Check sheet for the modelled part. Datum: model origin and axes. Units: mm. Face numbers are marked on the shaded views. A direction names the side the tool comes from. Round coordinates to 2 decimals unless told otherwise and drop trailing zeros. Order: outer loops, then holes, each group sorted by start corner. A loop starts at its lowest first (then second) coordinate and runs counter-clockwise, first axis right, second up. Notation, with made-up numbers: (-14, -26) -> (1, -26) arc R27 ccw to (1, 7) -> close; hole circle Ø10 at (29.5, -27). An arc over 180 degrees is marked (long way). Use CSV: the item, a comma, the result in double quotes.
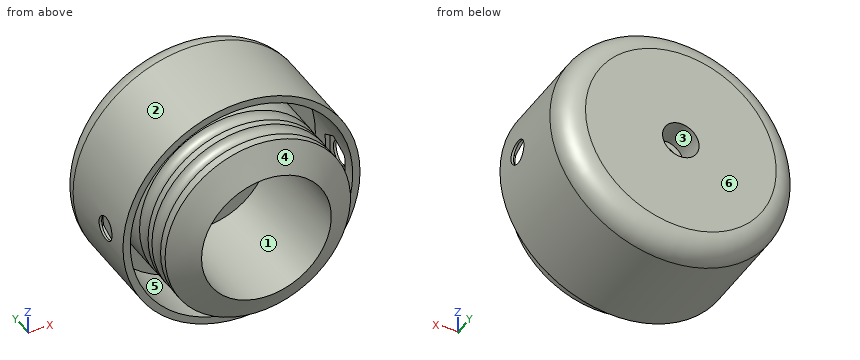
Autodesk Inventor part; units mm, degrees
ref_plane "Work Plane4" through (-32.48, 0, 0) normal (1, 0, 0) x (0, 1, 0)
ref_plane "Work Plane5" through (30.48, 0, 0) normal (1, 0, 0) x (0, 1, 0)
ref_plane "XZ Plane" through (0, 0, 0) normal (0, 1, 0) x (-1, 0, 0)
sketch "Sketch1" plane through (0, 0, 0) normal (0, 1, 0) x (-1, 0, 0)
  circle A0 centre (0, 0) radius 30.48
  circle A1 centre (0, 0) radius 32.48
  dimension "d0" = 60.96
  dimension "d2" = 2
extrude "Extrusion1" add sketch "Sketch1" along normal blind 19.05
sketch "Sketch2" plane through (0, 19.05, 0) normal (0, 1, 0) x (1, 0, 0)
  circle A0 centre (0, 0) radius 32.48
  circle A1 centre (0, 0) radius 32.48
extrude "Extrusion2" add sketch "Sketch2" along normal blind 12.7
fillet "Fillet1" radius 6.35 1 edges at (-32.48, 31.75, 0)
sketch "Sketch6" plane through (0, 31.75, 0) normal (0, 1, 0) x (1, 0, 0)
  circle A0 centre (0, 0) radius 3.302
  dimension "d15" = 6.604
extrude "Extrusion5" cut sketch "Sketch6" against normal up to surface (12.7 mm away)
sketch "Sketch10" plane through (0, 0, 0) normal (0, 0, 1) x (1, 0, 0)
  line L0 (-17.78, 19.05) -> (-17.78, -12.7)
  line L1 (-17.78, -12.7) -> (-25.4, -12.7)
  line L2 (-25.4, -12.7) -> (-25.4, 19.05)
  line L3 (-17.78, 19.05) -> (-25.4, 19.05)
  line L4 (-26.13, 31.75) -> (26.13, 31.75)
  line L5 (0, 31.75) -> (0, 0)
  line L6 (32.48, 0) -> (-32.48, 0)
  line L7 (-30.48, 0) -> (-30.48, 19.05)
  line L8 (-17.78, -12.7) -> (-25.4, -8.3006)
  line L9 (-30.48, 19.05) -> (30.48, 19.05)
  point P0 (-30.48, 0)
  point P1 (-25.4, 19.05)
  dimension "d29" = 7.62
  dimension "d33" = 30
  dimension "d42" = 25.4
  dimension "d89" = 31.75
revolve "Revolution2" add sketch "Sketch10" angle 360 about axis through (0, 31.75, 0) along (0, -1, 0) contours L0 L6 L2 L3 | L0 L8 L2 L6
sketch "Sketch11" plane through (0, 0, 0) normal (0, 0, 1) x (1, 0, 0)
  line L0 (25.4, -7.0306) -> (25.4, 25.4)
  circle A0 centre (26.3462, -3.81) radius 2.3813
  circle A1 centre (26.3462, 2.54) radius 2.3813
  line L1 (0, -11.43) -> (0, 31.75)
  line L2 (-26.13, 31.75) -> (26.13, 31.75)
  line L3 (26.3462, 2.54) -> (26.3462, -3.81)
  line L4 (30.48, 19.05) -> (30.48, 0)
  line L5 (30.48, 0) -> (29.972, 19.05)
  line L6 (29.972, 19.05) -> (29.972, 0)
  line L7 (-25.4, -5.08) -> (25.4, -5.08)
  line L8 (-17.78, -12.7) -> (17.78, -12.7)
  point P0 (0, 0)
  point P1 (25.4, -8.3006)
  point P2 (27.772, -0.6806)
  point P3 (17.78, -12.7)
  dimension "d36" = 6.35
  dimension "d37" = 4.7625
  dimension "d38" = 4.7625
  dimension "d43" = 26.3462
  dimension "d91" = 8.89
revolve "Revolution3" cut sketch "Sketch11" angle 360 about axis through (0, -11.43, 0) along (0, 1, 0) contours A0 L7 L0 | L0 A0 | L7 A0 L0 | A1 L0 | L0 A1
sketch "Sketch23" plane through (0, 31.75, 0) normal (0, 1, 0) x (1, 0, 0)
  circle A0 centre (0, 0) radius 5
  dimension "d103" = 10
extrude "Extrusion15" cut sketch "Sketch23" against normal blind 8
ref_plane "Work Plane4" through (-32.48, 0, 0) normal (1, 0, 0) x (0, 1, 0)
sketch "Sketch24" plane through (-32.48, 0, 0) normal (1, 0, 0) x (0, 1, 0)
  circle A0 centre (8.89, 0) radius 3.3
  line L0 (0, -32.48) -> (0, 32.48)
  line L1 (31.75, 5) -> (31.75, -5)
  line L2 (31.75, 0) -> (0, 0) construction
  line L3 (-1.6248, -25.4) -> (-1.6248, 25.4)
  dimension "d106" = 6.6
  dimension "d107" = 8.89
  dimension "d108" = 0
extrude "Extrusion16" cut sketch "Sketch24" along normal up to surface
pattern_circular "Circular Pattern4" count 2 over 360 about axis through (0, 31.75, 0) along (0, -1, 0) of "Extrusion16"
ref_plane "Work Plane5" through (30.48, 0, 0) normal (1, 0, 0) x (0, 1, 0)
sketch "Sketch25" plane through (30.48, 0, 0) normal (1, 0, 0) x (0, 1, 0)
  line L0 (31.75, 5) -> (31.75, -5)
  line L1 (31.75, 0) -> (-12.7, 0)
  line L2 (-12.7, 17.78) -> (-12.7, -17.78)
  line L3 (13.89, -2.8868) -> (8.89, -5.7735)
  line L4 (8.89, -5.7735) -> (3.89, -2.8868)
  line L5 (3.89, -2.8868) -> (3.89, 2.8868)
  line L6 (3.89, 2.8868) -> (8.89, 5.7735)
  line L7 (8.89, 5.7735) -> (13.89, 2.8868)
  line L8 (13.89, 2.8868) -> (13.89, -2.8868)
  line L9 (0, -32.48) -> (0, 32.48)
  circle A0 centre (8.89, 0) radius 1.45
  point P0 (0, 0)
  point P1 (13.89, 0)
  dimension "d115" = 8.89
  dimension "d116" = 2.9
  dimension "d117" = 10
extrude "Extrusion17" cut sketch "Sketch25" along normal blind 1.27 and the other way blind 0.635 contours L8 L3 L4 L5 L1 A0 | L1 A0 L5 L6 L7 L8
pattern_circular "Circular Pattern5" count 2 over 360 about axis through (0, 31.75, 0) along (0, -1, 0) of "Extrusion17"
properties part number "Water_Sensor_Cap_3DPrint"
Q1. Access from +Z, -Z, +X, -X, +Y, -Y to the whole of each face (thin tool, end or side, straight path). Record for the marked faces 1, 2 and 3.
Result sheet:
face 1,"-Y"
face 2,"+Y, -Y"
face 3,"+Y"
Q2. Mould release check, pull along X, two halves, no side actions. Record for the marked faces 4, 5 and 6: pulls with the +X half, pulls with the -X half, needs draft (parallel to the pull), parting line crosses it, or undercut.
Result sheet:
face 4,"parting line crosses it"
face 5,"undercut"
face 6,"needs draft"
Q3. Sectioned sample at C-C, the plane z = -24. State how many separate pieces and enclosed holes the cut face has, then the cut area to 3 significant figures.
Result sheet:
separate pieces,"3"
enclosed holes,"0"
area,"1,020 mm^2"
Q4. Go/stop test with flat-tipped pins: pin 1 (1.5 mm diameter, centred on x = 31.5, z = 0, fed in from -Y); pin 2 (1 mm diameter, centred on y = 4.5, z = 19, fed in from -X); pin 3 (1 mm diameter, centred on x = -15, y = 21, fed in from -Z); pin 4 (5.5 mm diameter, centred on x = 0, z = 0, fed in from -Y). Record where each tip stops, or that it passes through.
Result sheet:
pin 1,"stops at y = 0"
pin 2,"stops at x = -26.7"
pin 3,"stops at z = -29.06"
pin 4,"passes through"
Q5. Sectioned sample at D-D, the plane y = -5. Enter the section's corners in (x, z), then the cut area to 3 significant figures.
Result sheet:
outline,"circle Ø48.57 at (0, 0); hole circle Ø35.56 at (0, 0)"
area,"859 mm^2"
Q6. Scan lines: L1, parallel to X at y = 22.7, z = 0; L2, parallel to X at y = 6, z = -6; L3, parallel to X at y = 16.5, z = 22. Record each from-to range of solid material in increasing order.
Result sheet:
L1,"x = -32.48 to -3.3, 3.3 to 32.48"
L2,"x = -31.92 to -29.88, -24.68 to -16.74, 16.74 to 24.68, 29.88 to 31.92"
L3,"x = -23.89 to -21.1, -12.69 to 12.69, 21.1 to 23.89"
Q7. Sectioned sample at A-A, the plane y = 17. Enter the section's corners in (x, z), then the cut area to 3 significant figures.
Result sheet:
outline,"circle Ø64.96 at (0, 0); circle Ø50.8 at (0, 0); hole circle Ø60.96 at (0, 0); hole circle Ø35.56 at (0, 0)"
area,"1,430 mm^2"
